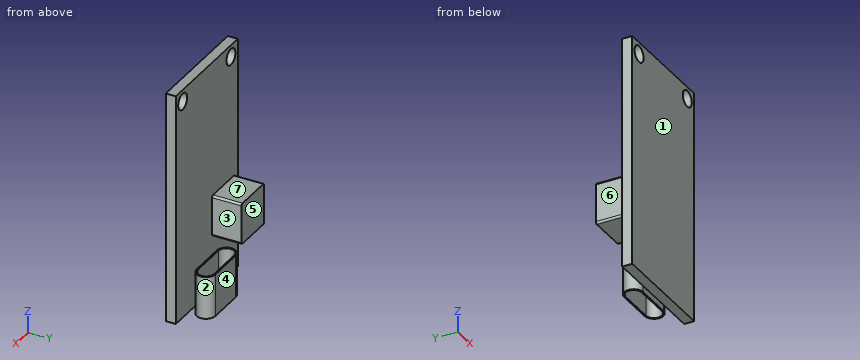
```python
from build123d import *

# Parameters (mm, degrees)
SKETCH1_W                = 18
SKETCH1_H                = 37.15
BOSS_EXTRUDE1_DEPTH      = 1.6
SKETCH2_R                = 1.3
CUT_EXTRUDE1_DEPTH       = 21.702430413
BOSS_EXTRUDE2_DEPTH      = 1
BOSS_EXTRUDE2_DEPTH_BACK = 5.8
SKETCH4_W                = 6.58
SKETCH4_H                = 6.58
BOSS_EXTRUDE3_DEPTH      = 4.72
FILLET1_R                = 0.3


with BuildPart() as part:
    # Sketch1 → Boss-Extrude1 (new body)
    with BuildSketch(Plane(origin=(0, 0, 0), x_dir=(1, 0, 0), z_dir=(0, 1, 0))):
        Rectangle(SKETCH1_W, SKETCH1_H)
    extrude(amount=BOSS_EXTRUDE1_DEPTH)

    # Sketch2 → Cut-Extrude1 (cut, through all)
    with BuildSketch(Plane(origin=(0, 1.6, 0), x_dir=(1, 0, 0), z_dir=(0, 1, 0))):
        with Locations(Location((-7, -16.675, 0), (0, 0, 270))):
            Circle(SKETCH2_R)
        with Locations(Location((7, -16.675, 0), (0, 0, 270))):
            Circle(SKETCH2_R)
    extrude(amount=-CUT_EXTRUDE1_DEPTH, mode=Mode.SUBTRACT)

    # Sketch3 → Boss-Extrude2 (add, two sides: drawn at the far end of the back side and taken through both)
    with BuildSketch(Plane(origin=(0, 0, -18.575), x_dir=(-1, 0, 0), z_dir=(0, 0, -1)).offset(-BOSS_EXTRUDE2_DEPTH_BACK)):
        with BuildLine():
            Line((2.93, 1.6), (-2.93, 1.6))
            ThreePointArc((-2.93, 1.6), (-4.43, 3.1), (-2.93, 4.6))
            Line((-2.93, 4.6), (2.93, 4.6))
            ThreePointArc((2.93, 4.6), (4.43, 3.1), (2.93, 1.6))
        make_face()
        with BuildLine():
            Line((2.93, 1.82), (-2.93, 1.82))
            ThreePointArc((-2.93, 1.82), (-4.21, 3.1), (-2.93, 4.38))
            Line((-2.93, 4.38), (2.93, 4.38))
            ThreePointArc((2.93, 4.38), (4.21, 3.1), (2.93, 1.82))
        make_face(mode=Mode.SUBTRACT)
    extrude(amount=BOSS_EXTRUDE2_DEPTH + BOSS_EXTRUDE2_DEPTH_BACK)

    # Sketch4 → Boss-Extrude3 (add)
    with BuildSketch(Plane(origin=(0, 1.6, 0), x_dir=(1, 0, 0), z_dir=(0, 1, 0))):
        with Locations((-4.81, 6.435)):
            Rectangle(SKETCH4_W, SKETCH4_H)
    extrude(amount=BOSS_EXTRUDE3_DEPTH)

    # Fillet1
    fillet1_edges = [part.edges().sort_by_distance(p)[0] for p in [
        (-1.52, 3.96, -3.145),
        (-1.52, 3.96, -9.725),
        (-8.1, 3.96, -9.725),
        (-8.1, 3.96, -3.145),
    ]]
    fillet(fillet1_edges, radius=FILLET1_R)


solid = part.part
```
The listing builds one solid part. Answer for the finished solid, in the listing's coordinates (mm). Face numbers are marked on the shaded views. A direction names the side the tool comes from. Give positions to 0.01 mm unless a question says otherwise; leave off trailing zeros. Order: outer loops, then holes, each group sorted by start corner. A loop starts at its lowest first (then second) coordinate and runs counter-clockwise, first axis right, second up. Notation, with made-up numbers: M 62,-22 L 121,-22 A17 cw 121,-1 Z; hole C 44,-28 d1. An arc over 180 degrees is marked long. Put each result on its own line as item: value. Start each with the question number.
Item 1: Which of the six approach directions +Z, -Z, +X, -X, +Y, -Y give full straight-line access (tool end or side, diameter ignored) to the marked faces 4, 5, 6 and 7?
Item 2: Find the intervals of material crossed by line 1 along Y through (x, z) = (1.25, -17); line 2 along Y through (x, z) = (-4, 5); line 3 along Z through (x, y) = (-3.5, 6.25) (3 decimals), in increasing order.
Item 3: The part is cut by section B-B, the plane z = -15. Determine the outline of the cut face in (x, y), and give its area (3 significant figures).
Item 4: For a pull along Y with two mould halves and no side action, classify the marked faces 1, 2 and 3 as +Y half, -Y half, draft (parallel to the pull), parting line (faces both ways), or undercut.
Item 5: Flat-ended cylindrical pins translate along their axes: P1, Ø3, axis at x = -1, z = -17, coming from the +Y side; P2, Ø3.5, axis at x = -0.5, y = 3.5, coming from the +Z side (3 decimals); P3, Ø2.5, axis at y = 5, z = -7.5, coming from the -X side. Find the tip coordinate at first contact, or state that the pin passes through.
Item 6: The part is cut by section C-C, the plane x = -7. Determine the outline of the cut face in (y, z) (3 decimals), and give its area (3 significant figures).
Item 7: The part is cut by section D-D, the plane y = 5.75. Determine the outline of the cut face in (x, z) (3 decimals).
Item 8: The part is cut by section A-A, the plane y = 3.1. Determine the outline of the cut face in (x, z) (3 decimals), and give its area (3 significant figures).
Answer key:
1. face 4: -Z, +X, -X, +Y
1. face 5: +Z, -Z, +X, -X, +Y
1. face 6: +Z, -Z, -X, +Y
1. face 7: +Z, +X, -X, +Y
2. line 1: y = 0 to 1.82, 4.38 to 4.6
2. line 2: y = 0 to 1.6
2. line 3: z = -9.725 to -3.145
3. outline: M -9,0 L 9,0 L 9,1.6 L 2.93,1.6 A1.5 ccw 2.93,4.6 L -2.93,4.6 A1.5 ccw -2.93,1.6 L -9,1.6 Z; hole M -2.93,1.82 L 2.93,1.82 A1.28 ccw 2.93,4.38 L -2.93,4.38 A1.28 ccw Z
3. area: 33.3 mm²
4. face 1: -Y half
4. face 2: undercut
4. face 3: draft
5. P1: stops at y = 4.6
5. P2: stops at z = -3.145
5. P3: stops at x = -8.1
6. outline: M 0,-18.575 L 1.6,-18.575 L 1.6,-9.725 L 6.32,-9.725 L 6.32,-3.145 L 1.6,-3.145 L 1.6,15.375 L 0,15.375 Z; M 0,17.975 L 1.6,17.975 L 1.6,18.575 L 0,18.575 Z
6. area: 86.3 mm²
7. outline: M -8.1,-9.425 A0.3 ccw -7.8,-9.725 L -1.82,-9.725 A0.3 ccw -1.52,-9.425 L -1.52,-3.445 A0.3 ccw -1.82,-3.145 L -7.8,-3.145 A0.3 ccw -8.1,-3.445 Z
8. outline: M -8.1,-9.425 A0.3 ccw -7.8,-9.725 L -1.82,-9.725 A0.3 ccw -1.52,-9.425 L -1.52,-3.445 A0.3 ccw -1.82,-3.145 L -7.8,-3.145 A0.3 ccw -8.1,-3.445 Z; M -4.43,-19.575 L -4.21,-19.575 L -4.21,-12.775 L -4.43,-12.775 Z; M 4.21,-19.575 L 4.43,-19.575 L 4.43,-12.775 L 4.21,-12.775 Z
8. area: 46.2 mm²
